```python
from build123d import *

# Parameters (mm, degrees)
SKETCH1_R           = 57.15
BOSS_EXTRUDE1_DEPTH = 20
SKETCH2_R           = 54.15
CUT_EXTRUDE1_DEPTH  = 14
BOSS_EXTRUDE2_DEPTH = 7
CUT_EXTRUDE2_DEPTH  = 84.260104492
SKETCH5_W           = 2
SKETCH5_H           = 16.000963959
CUT_EXTRUDE3_DEPTH  = 84.260104655
BOSS_EXTRUDE3_DEPTH = 18
BOSS_EXTRUDE4_DEPTH = 18
CUT_EXTRUDE4_DEPTH  = 9.75


with BuildPart() as part:
    # Sketch1 → Boss-Extrude1 (new body)
    with BuildSketch(Plane(origin=(0, 0, 0), x_dir=(1, 0, 0), z_dir=(0, 1, 0))):
        with Locations(Location((0, 0, 0), (0, 0, 270))):
            Circle(SKETCH1_R)
    extrude(amount=BOSS_EXTRUDE1_DEPTH)

    # Sketch2 → Cut-Extrude1 (cut)
    with BuildSketch(Plane(origin=(0, 20, 0), x_dir=(1, 0, 0), z_dir=(0, 1, 0))):
        with Locations(Location((0, 0, 0), (0, 0, 270))):
            Circle(SKETCH2_R)
    extrude(amount=-CUT_EXTRUDE1_DEPTH, mode=Mode.SUBTRACT)

    # Sketch3 → Boss-Extrude2 (add)
    with BuildSketch(Plane(origin=(0, 6, 0), x_dir=(1, 0, 0), z_dir=(0, 1, 0))):
        with BuildLine():
            ThreePointArc((-54.099007387, -2.349446691), (-51.8, 0), (-54.099007387, 2.349446691))
            ThreePointArc((-54.099007387, 2.349446691), (-54.15, 0), (-54.099007387, -2.349446691))
        make_face()
        with BuildLine():
            ThreePointArc((54.099007387, 2.349446691), (51.8, 0), (54.099007387, -2.349446691))
            ThreePointArc((54.099007387, -2.349446691), (54.15, 0), (54.099007387, 2.349446691))
        make_face()
    extrude(amount=BOSS_EXTRUDE2_DEPTH)

    # Sketch4 → Cut-Extrude2 (cut, through all)
    with BuildSketch(Plane.XY):
        with BuildLine():
            Line((2.75, 10.25), (2.75, 20))
            Line((2.75, 20), (-2.75, 20))
            Line((-2.75, 20), (-2.75, 10.25))
            ThreePointArc((-2.75, 10.25), (0, 7.5), (2.75, 10.25))
        make_face()
    extrude(amount=-CUT_EXTRUDE2_DEPTH, mode=Mode.SUBTRACT)

    # Sketch5 → Cut-Extrude3 (cut, through all)
    with BuildSketch(Plane.XY):
        with Locations((0.098176677, 11.999518021)):
            Rectangle(SKETCH5_W, SKETCH5_H)
    extrude(amount=CUT_EXTRUDE3_DEPTH, mode=Mode.SUBTRACT)

    # Sketch6 → Boss-Extrude3 (add)
    with BuildSketch(Plane.XY.offset(-54.15)):
        with BuildLine():
            Line((-4.25, 0), (4.25, 0))
            Line((4.25, 0), (4.25, 10.25))
            Line((4.25, 10.25), (2.75, 10.25))
            ThreePointArc((2.75, 10.25), (0, 7.5), (-2.75, 10.25))
            Line((-2.75, 10.25), (-4.25, 10.25))
            Line((-4.25, 10.25), (-4.25, 0))
        make_face()
    extrude(amount=-BOSS_EXTRUDE3_DEPTH)

    # Sketch7 → Boss-Extrude4 (add)
    with BuildSketch(Plane(origin=(0, 0, 54.15), x_dir=(-1, 0, 0), z_dir=(0, 0, -1))):
        with BuildLine():
            Line((4.25, 10.25), (1.5, 10.25))
            ThreePointArc((1.5, 10.25), (0, 8.75), (-1.5, 10.25))
            Line((-1.5, 10.25), (-4.25, 10.25))
            Line((-4.25, 10.25), (-4.25, 0))
            Line((-4.25, 0), (4.25, 0))
            Line((4.25, 0), (4.25, 10.25))
        make_face()
    extrude(amount=-BOSS_EXTRUDE4_DEPTH)

    # Sketch8 → Cut-Extrude4 (cut)
    with BuildSketch(Plane(origin=(0, 20, 0), x_dir=(1, 0, 0), z_dir=(0, 1, 0))):
        with BuildLine():
            Line((2.75, 54.080125739), (2.75, 57.083798052))
            Line((2.75, 57.083798052), (6.019401193, 53.814396859))
            ThreePointArc((6.019401193, 53.814396859), (4.386713152, 53.972022824), (2.75, 54.080125739))
        make_face()
        with BuildLine():
            Line((-2.75, 54.080125739), (-2.75, 57.083798052))
            Line((-2.75, 57.083798052), (-6.019401193, 53.814396859))
            ThreePointArc((-6.019401193, 53.814396859), (-4.386713152, 53.972022824), (-2.75, 54.080125739))
        make_face()
    extrude(amount=-CUT_EXTRUDE4_DEPTH, mode=Mode.SUBTRACT)


solid = part.part
```
Geometry: final body of the model. Coordinates: model frame, mm. A direction names the side the tool comes from. Coordinates: 2 decimals unless noted, no trailing zeros. Order: outer loops, then holes, each group sorted by start corner. A loop starts at its lowest first (then second) coordinate and runs counter-clockwise, first axis right, second up. Notation, with made-up numbers: (-33.5, 53.25) -> (15.5, 53.25) arc R18 cw to (15.5, 75.25) -> close; hole circle Ø5 at (42, -13.5). An arc over 180 degrees is marked (long way). Answer in a Markdown table with one row per item.
Item 1: Contact query for flat-ended pins moving along their axis: P1, Ø8, axis at x = -8.5, z = -45.5, coming from the +Y side; P2, Ø1, axis at x = 3.5, z = -55.5, coming from the +Y side; P3, Ø1, axis at y = 7.5, z = 22.5, coming from the -X side. Output: stop coordinate, or through.
Return value:
| item | result |
|---|---|
| P1 | stops at y = 6 |
| P2 | stops at y = 10.25 |
| P3 | stops at x = -52.75 |
Item 2: Section A-A on z = -63. Output: boundary loops of the cut face in (x, y), plus the area to 3 significant figures.
Return value:
| item | result |
|---|---|
| outline | (-4.25, 0) -> (4.25, 0) -> (4.25, 10.25) -> (2.75, 10.25) arc R2.75 cw to (-2.75, 10.25) -> (-4.25, 10.25) -> close |
| area | 75.2 mm² |
Item 3: Section C-C on y = 1.75. Output: boundary loops of the cut face in (x, z).
Return value:
| item | result |
|---|---|
| outline | (-4.25, -72.15) -> (4.25, -72.15) -> (4.25, -56.99) arc R57.15 ccw to (4.25, 56.99) -> (4.25, 72.15) -> (-4.25, 72.15) -> (-4.25, 56.99) arc R57.15 ccw to (-4.25, -56.99) -> close |
Item 4: Section B-B on x = 37.5. Output: boundary loops of the cut face in (y, z), plus the area to 3 significant figures.
Return value:
| item | result |
|---|---|
| outline | (0, -43.13) -> (20, -43.13) -> (20, -39.06) -> (6, -39.06) -> (6, 39.06) -> (20, 39.06) -> (20, 43.13) -> (0, 43.13) -> close |
| area | 631 mm² |
Item 5: Ray query, L1, parallel to X at y = 14, z = 0; L2, parallel to Y at x = -49, z = -16; L3, parallel to X at y = 12.25, z = -30. Return the intervals inside material, ascending.
Return value:
| item | result |
|---|---|
| L1 | x = -57.15 to -54.15, 54.15 to 57.15 |
| L2 | y = 0 to 6 |
| L3 | x = -48.64 to -45.08, 45.08 to 48.64 |
Item 6: Section D-D on z = 46. Output: boundary loops of the cut face in (x, y).
Return value:
| item | result |
|---|---|
| outline | (-33.91, 0) -> (33.91, 0) -> (33.91, 20) -> (28.57, 20) -> (28.57, 6) -> (1.1, 6) -> (1.1, 4) -> (-0.9, 4) -> (-0.9, 6) -> (-28.57, 6) -> (-28.57, 20) -> (-33.91, 20) -> close |
Item 7: Access query for faces 4 (the flat face through (4.25, 5, 64)), 5 (the flat face through (4.25, 5, -64)), 6 (the flat face through (4, 10.25, -55)). Directions: +Z, -Z, +X, -X, +Y, -Y. A direction counts if a zero-diameter tool reaches every point of the face in a straight line with its end or side. Return the directions, or none.
Return value:
| item | result |
|---|---|
| face 4 | +Z, +X, +Y, -Y |
| face 5 | -Z, +X, +Y, -Y |
| face 6 | +Y |
Item 8: Draft query along Z for faces 1 (the flat face through (0, 5, 72.15)), 2 (the cylindrical face through (-21.5, 13.1, 49.7)), 3 (the flat face through (-54, 20, 8)). Return one class per face: released by +Z, released by -Z, zero draft, split by the parting line, or undercut.
Return value:
| item | result |
|---|---|
| face 1 | released by +Z |
| face 2 | undercut |
| face 3 | zero draft |
